Print and shaded views of the part. All mm, measured from the part's lowest x, y and z. A direction names the side the tool comes from. Give positions to 0.01 mm unless a question says otherwise; leave off trailing zeros. Loops run counter-clockwise (first coordinate to the right, second up) from the corner with the lowest first, then second, coordinate; pieces in that order, holes last. Notation, with made-up numbers: (-24.5, -35.75) - (10.5, -35.75) arc R24 cw to (10.5, -18.75) - close; hole circle Ø3 at (52, 24). An arc over 180 degrees is marked (long way). Return JSON: item names as keys, results as strings.
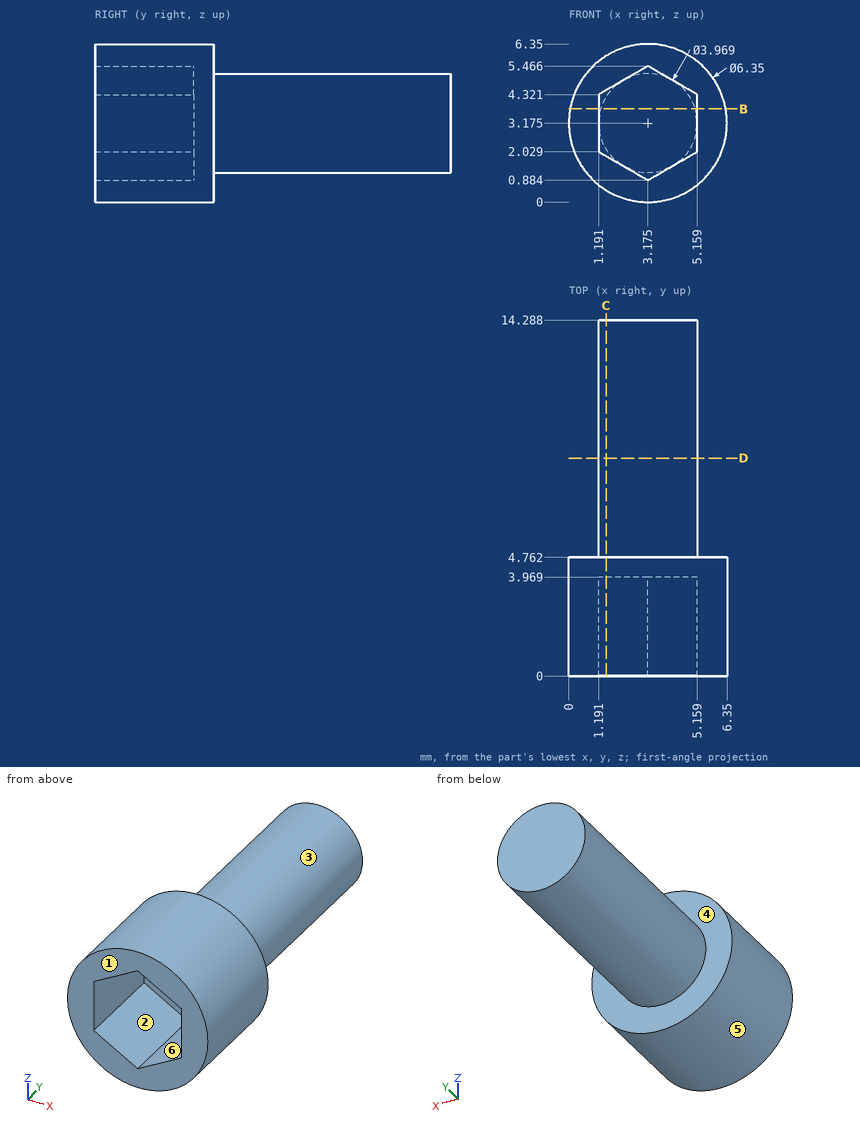
1. Pull direction Z, two halves, no side cores. Call the marked faces 1, 2 and 3: +Z half, -Z half, draft (parallel to the pull), parting line (faces both ways), or undercut.
Values follow:
{"face 1": "draft", "face 2": "undercut", "face 3": "parting line"}
2. Cut at D-D, the plane y = 8.75. Write the cut outline in (x, z) (1 decimal).
Values follow:
{"outline": "circle Ø4 at (3.2, 3.2)"}
3. Which spindle directions (+Z, -Z, +X, -X, +Y, -Y) get a long thin tool onto all of the face, cutting with end or side? Do the marked faces 4, 5 and 6. Say none if no direction does.
Values follow:
{"face 4": "+Y", "face 5": "+Y, -Y", "face 6": "-Y"}
4. Cut at B-B, the plane z = 3.75. Write the cut outline in (x, y) (1 decimal).
Values follow:
{"outline": "(0.1, 0) - (1.2, 0) - (1.2, 4) - (5.2, 4) - (5.2, 0) - (6.3, 0) - (6.3, 4.8) - (5.1, 4.8) - (5.1, 14.3) - (1.3, 14.3) - (1.3, 4.8) - (0.1, 4.8) - close"}
5. Drop flat-ended pins along their axis: P1, Ø2, axis at x = 4, y = 8.5, coming from the -Z side; P2, Ø2, axis at x = 5, y = 11.5, coming from the -Z side. Give the stop position or say it passes through.
Values follow:
{"P1": "stops at z = 1.19", "P2": "stops at z = 1.37"}
6. Drill centre lines: probe 1 along Y at (x, z) = (2.25, 2); probe 2 along Y at (x, z) = (5.25, 4.5); probe 3 along X at (y, z) = (2.5, 2.25). Where is each one in solid material? Low to high.
Values follow:
{"probe 1": "y = 3.97 to 14.29", "probe 2": "y = 0 to 4.76", "probe 3": "x = 0.14 to 1.19, 5.16 to 6.21"}
7. Cut at C-C, the plane x = 1.5. Write the cut outline in (y, z).
Values follow:
{"outline": "(0, 0.48) - (4.76, 0.48) - (4.76, 2.11) - (14.29, 2.11) - (14.29, 4.24) - (4.76, 4.24) - (4.76, 5.87) - (0, 5.87) - (0, 4.5) - (3.97, 4.5) - (3.97, 1.85) - (0, 1.85) - close"}
